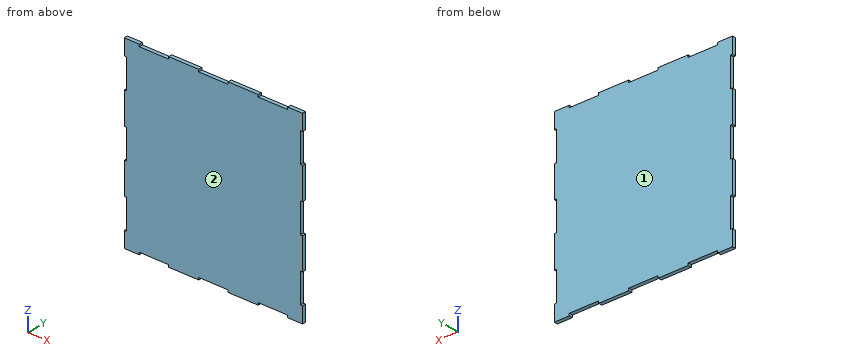
```python
from build123d import *

# Parameters (mm, degrees)
F1_DEPTH = 5


with BuildPart() as f1:
    # F0 (on Front) → F1 (new body)
    with BuildSketch(Plane.XZ):
        Polygon((100.7, -124), (121, -124), (121, -102.67), (118, -102.67), (118, -62.67), (121, -62.67), (121, -20), (118, -20), (118, 20), (121, 20), (121, 62.67), (118, 62.67), (118, 102.67), (121, 102.67), (121, 124), (100.7, 124), (100.7, 121), (60.7, 121), (60.7, 124), (20, 124), (20, 121), (-20, 121), (-20, 124), (-60.7, 124), (-60.7, 121), (-100.7, 121), (-100.7, 124), (-121, 124), (-121, 102.67), (-118, 102.67), (-118, 62.67), (-121, 62.67), (-121, 20), (-118, 20), (-118, -20), (-121, -20), (-121, -62.67), (-118, -62.67), (-118, -102.67), (-121, -102.67), (-121, -124), (-100.7, -124), (-100.7, -121), (-60.7, -121), (-60.7, -124), (-20, -124), (-20, -121), (20, -121), (20, -124), (60.7, -124), (60.7, -121), (100.7, -121), align=None)
    extrude(amount=F1_DEPTH)


solid = f1.part
```
Check sheet for the modelled part. Datum: model origin and axes. Units: mm. Face numbers are marked on the shaded views. Round coordinates to 2 decimals unless told otherwise and drop trailing zeros. Loops run counter-clockwise (first coordinate to the right, second up) from the corner with the lowest first, then second, coordinate; pieces in that order, holes last. Notation, with made-up numbers: (-19.75, 51.25) -> (9.25, 51.25) arc R9 ccw to (9.25, 62.25) -> close; hole circle Ø4 at (18, 64). An arc over 180 degrees is marked (long way). Write item = value, one per line. Start each with the question number.
1) Sectioned sample at B-B, the plane x = -72.5. Record the cut outline in (y, z).
2) Sectioned sample at A-A, the plane z = -97.5. Record the cut outline in (x, y).
3) Thickness scan on probe 1 along X at (y, z) = (-3, -17); probe 2 along Z at (x, y) = (-63, -1.8). Record the ranges inside material, lowest first.
4) Release check for a two-part mould opening along Y. For the marked faces 1 and 2 record: released by +Y, released by -Y, zero draft, split by the parting line, or undercut.
5) Gauge pin test, flat end, axial feed: pin 1 Ø2.5 at (x, y) = (7.5, -2) entering from -Z. Record the tip position at first contact, or that the pin passes through.
Results are:
q1.outline = (-5, -121) -> (0, -121) -> (0, 121) -> (-5, 121) -> close
q2.outline = (-118, -5) -> (118, -5) -> (118, 0) -> (-118, 0) -> close
q3.probe_1 = -118 to 118
q3.probe_2 = -121 to 121
q4.face_1 = released by +Y
q4.face_2 = released by -Y
q5.pin_1 = -121
